```python
from build123d import *

# Parameters (mm, degrees)
SKETCH2_W           = 24
SKETCH2_H           = 42
SKETCH2_W_2         = 7
SKETCH2_H_2         = 3.5
SKETCH2_W_3         = 2
BOSS_EXTRUDE1_DEPTH = 5
SKETCH2_3_W         = 7
SKETCH2_3_H         = 35
BOSS_EXTRUDE2_DEPTH = 2.5


with BuildPart() as part:
    # Sketch2 → Boss-Extrude1 (new body)
    with BuildSketch(Plane(origin=(0, 0, 0), x_dir=(1, 0, 0), z_dir=(0, 1, 0))):
        with Locations((14, 21)):
            Rectangle(SKETCH2_W, SKETCH2_H)
        Polygon((26, 42), (26, 0), (28, 0), (28, 3.5), (28, 38.5), (28, 42), align=None)
        with Locations((31.5, 1.75)):
            Rectangle(SKETCH2_W_2, SKETCH2_H_2)
        with BuildLine():
            Line((37, 42), (37, 0))
            Line((37, 0), (46, 0))
            ThreePointArc((46, 0), (49.535533906, 1.464466094), (51, 5))
            Line((51, 5), (51, 37))
            ThreePointArc((51, 37), (49.535533906, 40.535533906), (46, 42))
            Line((46, 42), (37, 42))
        make_face()
        with Locations((36, 21)):
            Rectangle(SKETCH2_W_3, SKETCH2_H)
        with Locations((31.5, 40.25)):
            Rectangle(SKETCH2_W_2, SKETCH2_H_2)
        with BuildLine():
            ThreePointArc((-23, 37), (-21.535533906, 40.535533906), (-18, 42))
            Line((-18, 42), (-9, 42))
            Line((-9, 42), (-9, 0))
            Line((-9, 0), (-18, 0))
            ThreePointArc((-18, 0), (-21.535533906, 1.464466094), (-23, 5))
            Line((-23, 5), (-23, 37))
        make_face()
        with Locations((-3.5, 1.75)):
            Rectangle(SKETCH2_W_2, SKETCH2_H_2)
        Polygon((-9, 42), (-9, 0), (-7, 0), (-7, 3.5), (-7, 38.5), (-7, 42), align=None)
        Polygon((0, 3.5), (0, 0), (2, 0), (2, 42), (0, 42), (0, 38.5), align=None)
        with Locations((-3.5, 40.25)):
            Rectangle(SKETCH2_W_2, SKETCH2_H_2)
        with BuildLine():
            Line((-13, -20), (41, -20))
            ThreePointArc((41, -20), (44.535533906, -18.535533906), (46, -15))
            Line((46, -15), (46, 0))
            Line((46, 0), (37, 0))
            Line((37, 0), (35, 0))
            Line((35, 0), (28, 0))
            Line((28, 0), (0, 0))
            Line((0, 0), (-7, 0))
            Line((-7, 0), (-9, 0))
            Line((-9, 0), (-18, 0))
            Line((-18, 0), (-18, -15))
            ThreePointArc((-18, -15), (-16.535533906, -18.535533906), (-13, -20))
        make_face()
        with BuildLine():
            Line((-13, 62), (41, 62))
            ThreePointArc((41, 62), (44.535533906, 60.535533906), (46, 57))
            Line((46, 57), (46, 42))
            Line((46, 42), (37, 42))
            Line((37, 42), (35, 42))
            Line((35, 42), (28, 42))
            Line((28, 42), (0, 42))
            Line((0, 42), (-7, 42))
            Line((-7, 42), (-9, 42))
            Line((-9, 42), (-18, 42))
            Line((-18, 42), (-18, 57))
            ThreePointArc((-18, 57), (-16.535533906, 60.535533906), (-13, 62))
        make_face()
    extrude(amount=BOSS_EXTRUDE1_DEPTH)

    # Sketch2_3 → Boss-Extrude2 (add)
    with BuildSketch(Plane(origin=(0, 0, 0), x_dir=(1, 0, 0), z_dir=(0, 1, 0))):
        with Locations((-3.5, 21)):
            Rectangle(SKETCH2_3_W, SKETCH2_3_H)
        with Locations((31.5, 21)):
            Rectangle(SKETCH2_3_W, SKETCH2_3_H)
    extrude(amount=BOSS_EXTRUDE2_DEPTH)


solid = part.part
```
Build history of the part. All positions in model axes, mm. A direction names the side the tool comes from. Give positions to 0.01 mm unless a question says otherwise; leave off trailing zeros. Loops run counter-clockwise (first coordinate to the right, second up) from the corner with the lowest first, then second, coordinate; pieces in that order, holes last.
Item 1: Slice it at C-C, the plane z = -13. List the corners of the cut face in (x, y).
Answers follow:
outline: (-23, 0) - (51, 0) - (51, 5) - (35, 5) - (35, 2.5) - (28, 2.5) - (28, 5) - (0, 5) - (0, 2.5) - (-7, 2.5) - (-7, 5) - (-23, 5) - close
Item 2: Slice it at B-B, the plane x = -2.5. List the corners of the cut face in (y, z).
Answers follow:
outline: (0, -62) - (5, -62) - (5, -38.5) - (2.5, -38.5) - (2.5, -3.5) - (5, -3.5) - (5, 20) - (0, 20) - close
Item 3: Which spindle directions (+Z, -Z, +X, -X, +Y, -Y) get a long thin tool onto all of the face, cutting with end or side? Do faces 1 (the face through (-23, 2, -21)), 2 (the face through (-18, 2, 7)), 3 (the face through (35, 4, -21)). Say none if no direction does.
Answers follow:
face 1: +Z, -Z, -X, +Y, -Y
face 2: +Z, -X, +Y, -Y
face 3: +Y
Item 4: Flat gauge pins, fed straight in: pin 1 (2.5 mm diameter, centred on y = 3.5, z = 7.5, fed in from -X); pin 2 (1 mm diameter, centred on x = -14, y = 1.5, fed in from -Z); pin 3 (1.5 mm diameter, centred on y = 2.5, z = 9.5, fed in from +X). Where does each tip first touch, or does it go through?
Answers follow:
pin 1: stops at x = -18
pin 2: stops at z = -61.97
pin 3: stops at x = 46
Item 5: Slice it at D-D, the plane z = 6.5. List the corners of the cut face in (x, y).
Answers follow:
outline: (-18, 0) - (46, 0) - (46, 5) - (-18, 5) - close
Item 6: Slice it at A-A, the plane y = 3.3. List the corners of the cut face in (x, z), and give its area (3 significant figures).
Answers follow:
outline: (-23, -37) arc R5 ccw to (-18, -42) - (-18, -57) arc R5 ccw to (-13, -62) - (41, -62) arc R5 ccw to (46, -57) - (46, -42) arc R5 ccw to (51, -37) - (51, -5) arc R5 ccw to (46, 0) - (46, 15) arc R5 ccw to (41, 20) - (-13, 20) arc R5 ccw to (-18, 15) - (-18, 0) arc R5 ccw to (-23, -5) - close; hole (-7, -38.5) - (0, -38.5) - (0, -3.5) - (-7, -3.5) - close; hole (28, -38.5) - (35, -38.5) - (35, -3.5) - (28, -3.5) - close
area: 5,140 mm2
Item 7: Drill centre lines: line 1 (X direction, y = 3.95, z = -22); line 2 (X direction, y = 3.85, z = -48.5); line 3 (Z direction, x = 34, y = 3.6). Where is each one in solid material? Low to high.
Answers follow:
line 1: x = -23 to -7, 0 to 28, 35 to 51
line 2: x = -18 to 46
line 3: z = -62 to -38.5, -3.5 to 20
Item 8: Pull direction X, two halves, no side cores. Call faces 4 (the face through (14, 2, 20)), 5 (the face through (0, 4, -21)), 6 (the face through (46, 2, 8)), 7 (the face through (-7, 4, -21)): released by +X, released by -X, zero draft, split by the parting line, or undercut.
Answers follow:
face 4: zero draft
face 5: undercut
face 6: released by +X
face 7: undercut
